from build123d import *

# Parameters (mm, degrees)
F0_R     = 4.7625
F1_DEPTH = 12.7
F3_D     = 3.4544
F3_DEPTH = 3.175
F3_TIP   = 1.0378064612
F4_D     = 3.4544
F4_DEPTH = 3.175
F4_TIP   = 1.0378064612


with BuildPart() as f1:
    # F0 (on Top) → F1 (new body)
    with BuildSketch(Plane.XY):
        with Locations((0, -0.0934494074)):
            Circle(F0_R)
    extrude(amount=F1_DEPTH)

    # F3
    with Locations(Plane.XY.offset(12.7)):
        with Locations((0, 0)):
            Hole(F3_D / 2, depth=F3_DEPTH)
            with Locations((0, 0, -(F3_DEPTH + F3_TIP / 2))):  # 118° drill point
                Cone(0, F3_D / 2, F3_TIP, mode=Mode.SUBTRACT)

    # F4
    with Locations(Plane(origin=(0, 0, 0), x_dir=(1, 0, 0), z_dir=(0, 0, -1))):
        with Locations((0, 0.0934494074)):
            Hole(F4_D / 2, depth=F4_DEPTH)
            with Locations((0, 0, -(F4_DEPTH + F4_TIP / 2))):  # 118° drill point
                Cone(0, F4_D / 2, F4_TIP, mode=Mode.SUBTRACT)


solid = f1.part
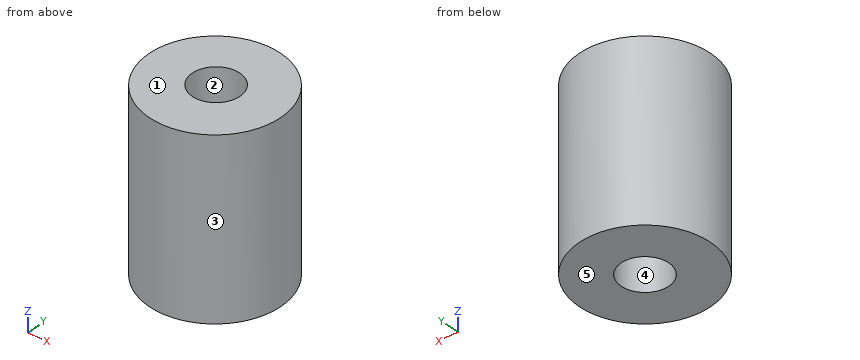
Source: CAD feature listing. Evaluate the final solid. Frame: model axes, mm. Face numbers are marked on the shaded views. A direction names the side the tool comes from. Round coordinates to 2 decimals unless told otherwise and drop trailing zeros. Loops run counter-clockwise (first coordinate to the right, second up) from the corner with the lowest first, then second, coordinate; pieces in that order, holes last. Notation, with made-up numbers: M 14.5,28 L 38.5,28 A31 cw 38.5,56 Z; hole C 6,20.5 d7. An arc over 180 degrees is marked long. Return JSON: item names as keys, results as strings. Group by question number.
1. Section query C-C on x = -3. Output: boundary loops of the cut face in (y, z), and give its area (3 significant figures).
2. Section query A-A on z = 10. Output: boundary loops of the cut face in (x, y) (1 decimal), and give its area (3 significant figures).
3. Pin query (flat end, axial travel): pin 1 (3 mm diameter, centred on x = 2, z = 6, fed in from -Y); pin 2 (1 mm diameter, centred on x = -2.5, z = 2.5, fed in from -Y); pin 3 (1.5 mm diameter, centred on x = -1, z = 5.5, fed in from +Y). Return the tip coordinate at first contact, or that it passes through.
4. Material intervals for line 1 along Y through (x, z) = (0, 2.3); line 2 along X through (y, z) = (-0.75, 3); line 3 along Y through (x, z) = (0.5, 1.5), sorted ascending. Write a range as from..to.
5. Section query B-B on y = -2.5. Output: boundary loops of the cut face in (x, z).
6. Reachability of the marked faces 4 and 5 from +Z, -Z, +X, -X, +Y, -Y: full face, straight path, thin tool, end or side. Return the list, or none.
7. Mould query, pull axis Y, two halves, no side actions, for the marked faces 1, 2 and 3. Classes: released by +Y, released by -Y, zero draft, split by the parting line, or undercut.
Checks:
{
 "1": {"outline": "M -3.79,0 L 3.61,0 L 3.61,12.7 L -3.79,12.7 Z", "area": "94.0 mm²"},
 "2": {"outline": "C 0,-0.1 d9.5; hole C 0,0 d3.5", "area": "61.9 mm²"},
 "3": {"pin 1": "stops at y = -4.83", "pin 2": "stops at y = -4.42", "pin 3": "stops at y = 4.66"},
 "4": {"line 1": "y = -4.86..-1.82, 1.63..4.67", "line 2": "x = -4.72..-1.6, 1.6..4.72", "line 3": "y = -4.83..-1.75, 1.56..4.64"},
 "5": {"outline": "M -4.11,0 L 4.11,0 L 4.11,12.7 L -4.11,12.7 Z"},
 "6": {"face 4": "-Z", "face 5": "-Z, +X, -X, +Y, -Y"},
 "7": {"face 1": "zero draft", "face 2": "undercut", "face 3": "split by the parting line"}
}
